For this review, take the finished solid that the model builds, in its own axes (mm). Face numbers are marked on the shaded views. Round coordinates to 2 decimals unless told otherwise and drop trailing zeros. Write each loop counter-clockwise with the first axis right and the second up, starting at its lowest first coordinate (ties: lowest second). Pieces come first, ordered by that corner, then holes. Notation, with made-up numbers: (-34, 73) -> (-13, 73) arc R28 ccw to (-13, 96) -> close; hole circle Ø3 at (-18, 2.25). An arc over 180 degrees is marked (long way). Answer as CSV lines item,"result". Start each with the question number.
Item 1: Take a section at A-A on z = -3. Give the boundary of the cut face in (x, y), then the cut area to 3 significant figures.
Item 2: Take a section at B-B on x = -3. Give the boundary of the cut face in (y, z).
Item 3: Wall thickness on probe 1 along Z at (x, y) = (-12, -3.8); probe 2 along X at (y, z) = (-2.3, 7): over which ranges is each line inside the solid? List them lowest first. Write a range as from..to.
Item 4: For pin 1 Ø1 at (y, z) = (-3.5, 24.5) entering from -X; pin 2 Ø1.5 at (x, z) = (1, -0.5) entering from -Y; pin 3 Ø1.5 at (y, z) = (-1.5, 0) entering from +X, all flat-tipped, find the tip position at first contact; note any pin that passes through.
Item 5: Mouldability with a two-part tool opening along X and no side actions: class the marked faces 1 and 2 as +X half, -X half, draft (parallel to the pull), parting line (faces both ways), or undercut.
```python
from build123d import *

# Parameters (mm, degrees)
F1_DEPTH = 4.5
F2_DEPTH = 3.5
F3_DEPTH = 1
F4_R     = 2.5


with BuildPart() as f1:
    # F0 (on Front) → F1 (new body)
    with BuildSketch(Plane.XZ):
        with BuildLine():
            Line((15.95, 30.95), (-15.95, 30.95))
            ThreePointArc((-15.95, 30.95), (-26.556602, 26.556602), (-30.95, 15.95))
            Line((-30.95, 15.95), (-30.95, -15.95))
            ThreePointArc((-30.95, -15.95), (-26.556602, -26.556602), (-15.95, -30.95))
            Line((-15.95, -30.95), (15.95, -30.95))
            ThreePointArc((15.95, -30.95), (26.556602, -26.556602), (30.95, -15.95))
            Line((30.95, -15.95), (30.95, 15.95))
            ThreePointArc((30.95, 15.95), (26.556602, 26.556602), (15.95, 30.95))
        make_face()
        with BuildLine():
            ThreePointArc((-29.949999, 15.95), (-25.849494, 25.849494), (-15.95, 29.949999))
            Line((-15.95, 29.949999), (15.95, 29.949999))
            ThreePointArc((15.95, 29.949999), (25.849494, 25.849494), (29.949999, 15.95))
            Line((29.949999, 15.95), (29.949999, -15.95))
            ThreePointArc((29.949999, -15.95), (25.849494, -25.849494), (15.95, -29.949999))
            Line((15.95, -29.949999), (-15.95, -29.949999))
            ThreePointArc((-15.95, -29.949999), (-25.849494, -25.849494), (-29.949999, -15.95))
            Line((-29.949999, -15.95), (-29.949999, 15.95))
        make_face(mode=Mode.SUBTRACT)
    extrude(amount=F1_DEPTH)

    # F0 (on Front) → F2 (join)
    with BuildSketch(Plane.XZ):
        with BuildLine():
            Line((15.95, 29.949999), (-15.95, 29.949999))
            ThreePointArc((-15.95, 29.949999), (-25.849494, 25.849494), (-29.949999, 15.95))
            Line((-29.949999, 15.95), (-29.949999, -15.95))
            ThreePointArc((-29.949999, -15.95), (-25.849494, -25.849494), (-15.95, -29.949999))
            Line((-15.95, -29.949999), (15.95, -29.949999))
            ThreePointArc((15.95, -29.949999), (25.849494, -25.849494), (29.949999, -15.95))
            Line((29.949999, -15.95), (29.949999, 15.95))
            ThreePointArc((29.949999, 15.95), (25.849494, 25.849494), (15.95, 29.949999))
        make_face()
        with BuildLine():
            ThreePointArc((-29.45, 15.95), (-25.495942, 25.495942), (-15.95, 29.45))
            Line((-15.95, 29.45), (15.95, 29.45))
            ThreePointArc((15.95, 29.45), (25.495942, 25.495942), (29.45, 15.95))
            Line((29.45, 15.95), (29.45, -15.95))
            ThreePointArc((29.45, -15.95), (25.495942, -25.495942), (15.95, -29.45))
            Line((15.95, -29.45), (-15.95, -29.45))
            ThreePointArc((-15.95, -29.45), (-25.495942, -25.495942), (-29.45, -15.95))
            Line((-29.45, -15.95), (-29.45, 15.95))
        make_face(mode=Mode.SUBTRACT)
    extrude(amount=F2_DEPTH)

    # F0 (on Front) → F3 (join)
    with BuildSketch(Plane.XZ):
        with BuildLine():
            Line((15.95, 29.45), (-15.95, 29.45))
            ThreePointArc((-15.95, 29.45), (-25.495942, 25.495942), (-29.45, 15.95))
            Line((-29.45, 15.95), (-29.45, -15.95))
            ThreePointArc((-29.45, -15.95), (-25.495942, -25.495942), (-15.95, -29.45))
            Line((-15.95, -29.45), (15.95, -29.45))
            ThreePointArc((15.95, -29.45), (25.495942, -25.495942), (29.45, -15.95))
            Line((29.45, -15.95), (29.45, 15.95))
            ThreePointArc((29.45, 15.95), (25.495942, 25.495942), (15.95, 29.45))
        make_face()
    extrude(amount=F3_DEPTH)

    # F4
    f4_edges = [f1.edges().sort_by_distance(p)[0] for p in [
        (30.95, 0, 0),
    ]]
    fillet(f4_edges, radius=F4_R)


solid = f1.part
```
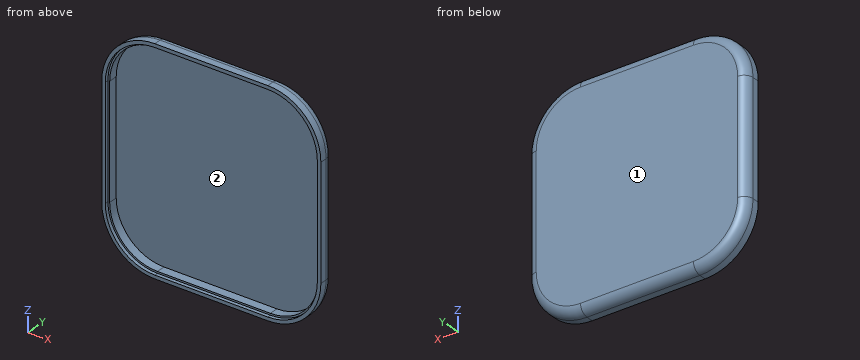
Output values:
1,outline,"(-30.95, -4.5) -> (-29.95, -4.5) -> (-29.95, -3.5) -> (-29.45, -3.5) -> (-29.45, -1) -> (29.45, -1) -> (29.45, -3.5) -> (29.95, -3.5) -> (29.95, -4.5) -> (30.95, -4.5) -> (30.95, -2.5) arc R2.5 ccw to (28.45, 0) -> (-28.45, 0) arc R2.5 ccw to (-30.95, -2.5) -> close"
1,area,"68.7 mm^2"
2,outline,"(-4.5, -30.95) -> (-2.5, -30.95) arc R2.5 ccw to (0, -28.45) -> (0, 28.45) arc R2.5 ccw to (-2.5, 30.95) -> (-4.5, 30.95) -> (-4.5, 29.95) -> (-3.5, 29.95) -> (-3.5, 29.45) -> (-1, 29.45) -> (-1, -29.45) -> (-3.5, -29.45) -> (-3.5, -29.95) -> (-4.5, -29.95) -> close"
3,probe 1,"z = -30.95..-29.95, 29.95..30.95"
3,probe 2,"x = -30.94..-29.45, 29.45..30.94"
4,pin 1,"stops at x = -28.61"
4,pin 2,"stops at y = -1"
4,pin 3,"stops at x = 30.94"
5,face 1,"draft"
5,face 2,"undercut"
